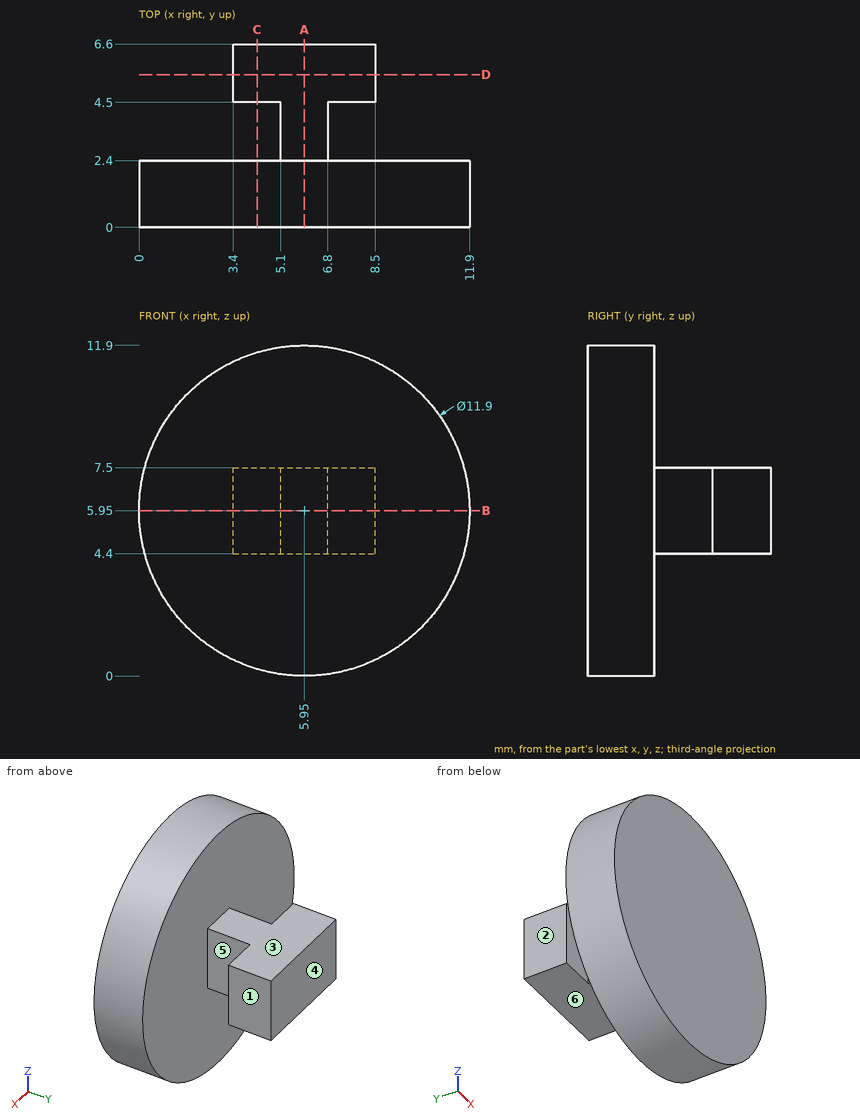
Geometry: see drawing. Coordinates: mm, zero at the bounding-box minimum. A direction names the side the tool comes from. Round coordinates to 2 decimals unless told otherwise and drop trailing zeros. Write each loop counter-clockwise with the first axis right and the second up, starting at its lowest first coordinate (ties: lowest second). Pieces come first, ordered by that corner, then holes. Notation, with made-up numbers: M 52,-8 L 105,-8 A23 cw 105,18 Z; hole C -21,34.5 d10. An arc over 180 degrees is marked long. Answer as a JSON object with one key per item and string values. Group by question number.
(1) Ray query, line 1 (Y direction, x = 9.75, z = 6); line 2 (Z direction, x = 6.25, y = 4.5); line 3 (Z direction, x = 1, y = 2). Return the intervals inside material, ascending. Write a range as [from, to].
(2) Section query C-C on x = 4.25. Output: boundary loops of the cut face in (y, z).
(3) Section query B-B on z = 5.95. Output: boundary loops of the cut face in (x, y), then the cut area to 3 significant figures.
(4) Section query A-A on x = 5.95. Output: boundary loops of the cut face in (y, z).
(5) Section query D-D on y = 5.5. Output: boundary loops of the cut face in (x, z).
(6) First-contact query: pin 1 (2 mm diameter, centred on y = 1.5, z = 3, fed in from -X); pin 2 (1 mm diameter, centred on y = 5.5, z = 6, fed in from -X); pin 3 (2.5 mm diameter, centred on y = 6, z = 6.5, fed in from +X). Flat tips, straight axial feed; report the tip coordinate or a pass-through.
(7) Reachability of the marked faces 1, 2 and 3 from +Z, -Z, +X, -X, +Y, -Y: full face, straight path, thin tool, end or side. Return the list, or none.
(8) Mould query, pull axis Y, two halves, no side actions, for the marked faces 4, 5 and 6. Classes: +Y half, -Y half, draft (parallel to the pull), parting line (faces both ways), or undercut.
Computed values:
{
 "1": {"line 1": "[0, 2.4]", "line 2": "[4.4, 7.5]", "line 3": "[2.65, 9.25]"},
 "2": {"outline": "M 0,0.25 L 2.4,0.25 L 2.4,11.65 L 0,11.65 Z; M 4.5,4.4 L 6.6,4.4 L 6.6,7.5 L 4.5,7.5 Z"},
 "3": {"outline": "M 0,0 L 11.9,0 L 11.9,2.4 L 6.8,2.4 L 6.8,4.5 L 8.5,4.5 L 8.5,6.6 L 3.4,6.6 L 3.4,4.5 L 5.1,4.5 L 5.1,2.4 L 0,2.4 Z", "area": "42.8 mm^2"},
 "4": {"outline": "M 0,0 L 2.4,0 L 2.4,4.4 L 6.6,4.4 L 6.6,7.5 L 2.4,7.5 L 2.4,11.9 L 0,11.9 Z"},
 "5": {"outline": "M 3.4,4.4 L 8.5,4.4 L 8.5,7.5 L 3.4,7.5 Z"},
 "6": {"pin 1": "x = 0.33", "pin 2": "x = 3.4", "pin 3": "x = 8.5"},
 "7": {"face 1": "+Z, -Z, +X, +Y", "face 2": "+Z, -Z, -X, +Y", "face 3": "+Z, +X, -X, +Y"},
 "8": {"face 4": "+Y half", "face 5": "undercut", "face 6": "draft"}
}
